from build123d import *

# Parameters (mm, degrees)
ESQUISSE1_R             = 57.5
ESQUISSE1_R_2           = 47.5
BOSS_EXTRU_1_DEPTH      = 30
ESQUISSE3_R             = 2.5
BOSS_EXTRU_3_DEPTH      = 40
ESQUISSE23_R            = 2.5
ENL_V_MAT_EXTRU_1_DEPTH = 10
ESQUISSE22_R            = 2.5
ENL_V_MAT_EXTRU_2_DEPTH = 10
ESQUISSE20_R            = 2.5
ENL_V_MAT_EXTRU_3_DEPTH = 10


with BuildPart() as part:
    # Esquisse1 → Boss.-Extru.1 (new body)
    with BuildSketch(Plane(origin=(0, 0, 0), x_dir=(1, 0, 0), z_dir=(0, 1, 0))):
        with Locations(Location((0, 0, 0), (0, 0, 270))):
            Circle(ESQUISSE1_R)
        with Locations(Location((0, 0, 0), (0, 0, 270))):
            Circle(ESQUISSE1_R_2, mode=Mode.SUBTRACT)
    extrude(amount=BOSS_EXTRU_1_DEPTH)

    # Esquisse3 → Boss.-Extru.3 (add)
    with BuildSketch(Plane(origin=(0, 0, 0), x_dir=(1, 0, 0), z_dir=(0, 1, 0))):
        with Locations(Location((0, 52.5, 0), (0, 0, 270))):
            Circle(ESQUISSE3_R)
        with Locations(Location((0, -52.5, 0), (0, 0, 270))):
            Circle(ESQUISSE3_R)
        with Locations(Location((-52.5, 0, 0), (0, 0, 270))):
            Circle(ESQUISSE3_R)
        with Locations(Location((52.5, 0, 0), (0, 0, 270))):
            Circle(ESQUISSE3_R)
    extrude(amount=BOSS_EXTRU_3_DEPTH)

    # Esquisse23 → Enlèv. mat.-Extru.1 (cut)
    with BuildSketch(Plane(origin=(0, 0, 0), x_dir=(1, 0, 0), z_dir=(0, 1, 0))):
        with Locations(Location((52.5, 0, 0), (0, 0, 270))):
            Circle(ESQUISSE23_R)
    extrude(amount=ENL_V_MAT_EXTRU_1_DEPTH, mode=Mode.SUBTRACT)

    # Esquisse22 → Enlèv. mat.-Extru.2 (cut)
    with BuildSketch(Plane(origin=(0, 0, 0), x_dir=(1, 0, 0), z_dir=(0, 1, 0))):
        with Locations(Location((0, 52.5, 0), (0, 0, 270))):
            Circle(ESQUISSE22_R)
    extrude(amount=ENL_V_MAT_EXTRU_2_DEPTH, mode=Mode.SUBTRACT)

    # Esquisse20 → Enlèv. mat.-Extru.3 (cut)
    with BuildSketch(Plane(origin=(0, 0, 0), x_dir=(1, 0, 0), z_dir=(0, 1, 0))):
        with Locations(Location((0, -52.5, 0), (0, 0, 270))):
            Circle(ESQUISSE20_R)
        with Locations(Location((-52.5, 0, 0), (0, 0, 270))):
            Circle(ESQUISSE20_R)
        with Locations(Location((0, 52.5, 0), (0, 0, 270))):
            Circle(ESQUISSE20_R)
        with Locations(Location((52.5, 0, 0), (0, 0, 270))):
            Circle(ESQUISSE20_R)
    extrude(amount=ENL_V_MAT_EXTRU_3_DEPTH, mode=Mode.SUBTRACT)


solid = part.part
Can you work these out from the model? Positions are in its coordinate system, mm. A direction names the side the tool comes from. Give positions to 0.01 mm unless a question says otherwise; leave off trailing zeros. Loops run counter-clockwise (first coordinate to the right, second up) from the corner with the lowest first, then second, coordinate; pieces in that order, holes last. Notation, with made-up numbers: M -0.75,-1.75 L 40.25,-1.75 A20 ccw 40.25,21.25 Z; hole C 87.25,87.5 d7. An arc over 180 degrees is marked long. One line per item, written item: value. Start each with the question number.
1) If we section it at C-C, the plane y = 11.5: Write out the boundary of the cut face in (x, z), and give its area (3 significant figures).
2) If we section it at D-D, the plane x = 52.5: Write out the boundary of the cut face in (y, z).
3) If we section it at A-A, the plane x = 0: Write out the boundary of the cut face in (y, z), and give its area (3 significant figures).
4) I'm going to push flat-ended pins straight in: pin 1 (2.5 mm diameter, centred on x = 52.5, z = -0.5, fed in from -Y); pin 2 (5 mm diameter, centred on x = -37.5, y = 22, fed in from -Z); pin 3 (2 mm diameter, centred on x = -13, y = 7, fed in from -Z); pin 4 (4 mm diameter, centred on x = 34, z = -28, fed in from -Y). Where does each tip first touch, or does it pass through?
5) On a 3-axis mill with a long thin cutter (end or side, diameter ignored), from which of +Z, -Z, +X, -X, +Y, -Y can I reach the whole of each face in a straight line? I mean faces 1 (the face through (-54.94, 4.93, -0.54)), 2 (the face through (-0.96, 34.93, -50.19)), 3 (the face through (-52, 40, 0)). Say none if no direction works.
6) If I drill on line 1 (X direction, y = 3, z = 0); line 2 (X direction, y = 18, z = -0.5); line 3 (Z direction, x = -17, y = 12.5), over which ranges is the centre line in solid material (lowest first)? Write a range as [from, to].
7) Thinking about a two-plate mould opening in X: for faces 4 (the face through (-54.94, 34.93, -0.54)), 5 (the face through (-56.133, 14.79, -12.465)), 6 (the face through (0, 40, -53)), 7 (the face through (50.06, 4.93, -0.54)), which applies, +X half, -X half, draft (parallel to the pull), parting line (faces both ways), or undercut?
8) If we section it at B-B, the plane z = 0: Write out the boundary of the cut face in (x, y), and give its area (3 significant figures).
Completed:
1. outline: C 0,0 d115; hole C 0,0 d95
1. area: 3,300 mm^2
2. outline: M 0,-23.45 L 30,-23.45 L 30,-2.5 L 40,-2.5 L 40,2.5 L 30,2.5 L 30,23.45 L 0,23.45 L 0,2.5 L 10,2.5 L 10,-2.5 L 0,-2.5 Z
3. outline: M 0,-57.5 L 30,-57.5 L 30,-55 L 40,-55 L 40,-50 L 30,-50 L 30,-47.5 L 0,-47.5 L 0,-50 L 10,-50 L 10,-55 L 0,-55 Z; M 0,47.5 L 30,47.5 L 30,50 L 40,50 L 40,55 L 30,55 L 30,57.5 L 0,57.5 L 0,55 L 10,55 L 10,50 L 0,50 Z
3. area: 600 mm^2
4. pin 1: stops at y = 10
4. pin 2: stops at z = -45.62
4. pin 3: stops at z = -56.23
4. pin 4: passes through
5. face 1: -Y
5. face 2: +Y
5. face 3: +Z, -Z, +X, -X, +Y
6. line 1: x = [-57.5, -55], [-50, -47.5], [47.5, 50], [55, 57.5]
6. line 2: x = [-57.5, -47.5], [47.5, 57.5]
6. line 3: z = [-54.93, -44.35], [44.35, 54.93]
7. face 4: undercut
7. face 5: parting line
7. face 6: draft
7. face 7: undercut
8. outline: M -57.5,0 L -55,0 L -55,10 L -50,10 L -50,0 L -47.5,0 L -47.5,30 L -50,30 L -50,40 L -55,40 L -55,30 L -57.5,30 Z; M 47.5,0 L 50,0 L 50,10 L 55,10 L 55,0 L 57.5,0 L 57.5,30 L 55,30 L 55,40 L 50,40 L 50,30 L 47.5,30 Z
8. area: 600 mm^2
